```python
from build123d import *

# Parameters (mm, degrees)
SKETCH1_W           = 50.8
SKETCH1_H           = 65.000000038
SKETCH1_R           = 2.5
EXTRUDE_5_DEPTH     = 7.5
SKETCH1_3_W         = 50.8
SKETCH1_3_H         = 10
BOSS_EXTRUDE1_DEPTH = 34.125
BOSS_EXTRUDE2_START = 34.125
BOSS_EXTRUDE2_DEPTH = 5
CHAMFER1_SIZE       = 10
CHAMFER1_SIZE2      = 27.474774195
FILLET1_R           = 3
SKETCH2_R           = 5
CUT_EXTRUDE1_DEPTH  = 144.721138443
SKETCH3_R           = 2.5
CUT_EXTRUDE2_DEPTH  = 144.721138443
SKETCH4_R           = 3.55
CUT_EXTRUDE3_DEPTH  = 4
SKETCH5_R           = 3.55
CUT_EXTRUDE4_DEPTH  = 4
BOSS_EXTRUDE3_START = -3.18
SKETCH1_5_W         = 50.8
SKETCH1_5_H         = 10
SKETCH1_5_H_2       = 65.000000038
SKETCH1_5_R         = 2.5
BOSS_EXTRUDE3_DEPTH = 3.18


with BuildPart() as part:
    # Sketch1 → 5 (new body)
    with BuildSketch(Plane.XY):
        with Locations((0, 102.500000019)):
            Rectangle(SKETCH1_W, SKETCH1_H)
        with Locations((-11.25, 85.000000038)):
            Circle(SKETCH1_R, mode=Mode.SUBTRACT)
        with Locations((-11.25, 120.000000038)):
            Circle(SKETCH1_R, mode=Mode.SUBTRACT)
        with Locations((11.25, 85.000000038)):
            Circle(SKETCH1_R, mode=Mode.SUBTRACT)
        with Locations((11.25, 120.000000038)):
            Circle(SKETCH1_R, mode=Mode.SUBTRACT)
    extrude(amount=EXTRUDE_5_DEPTH)

    # Sketch1<3> → Boss-Extrude1 (add)
    with BuildSketch(Plane.XY):
        with Locations((0, 65)):
            Rectangle(SKETCH1_3_W, SKETCH1_3_H)
    extrude(amount=BOSS_EXTRUDE1_DEPTH)

    # Sketch1<4> → Boss-Extrude2 (add)
    with BuildSketch(Plane.XY.offset(BOSS_EXTRUDE2_START)):
        with BuildLine():
            Line((-25.4, 70), (-25.4, 60))
            Line((-25.4, 60), (-26, 60))
            ThreePointArc((-26, 60), (-28.828427125, 58.828427125), (-30, 56))
            Line((-30, 56), (-30, 4))
            ThreePointArc((-30, 4), (-28.828427125, 1.171572875), (-26, 0))
            Line((-26, 0), (26, 0))
            ThreePointArc((26, 0), (28.828427125, 1.171572875), (30, 4))
            Line((30, 4), (30, 56))
            ThreePointArc((30, 56), (28.828427125, 58.828427125), (26, 60))
            Line((26, 60), (25.4, 60))
            Line((25.4, 60), (25.4, 70))
            Line((25.4, 70), (-25.4, 70))
        make_face()
    extrude(amount=BOSS_EXTRUDE2_DEPTH)

    # Chamfer1
    chamfer1_edges = [part.edges().sort_by_distance(p)[0] for p in [
        (0, 70, 7.5),
    ]]
    chamfer1_side = [part.faces().sort_by_distance(p)[0] for p in [
        (0, 102.500000019, 7.5),
    ]]
    chamfer(chamfer1_edges, length=CHAMFER1_SIZE, length2=CHAMFER1_SIZE2, reference=chamfer1_side[0])

    # Fillet1
    fillet1_edges = [part.edges().sort_by_distance(p)[0] for p in [
        (0, 70, 39.125),
        (0, 70, 34.974774195),
    ]]
    fillet(fillet1_edges, radius=FILLET1_R)

    # Sketch2 → Cut-Extrude1 (cut, through all)
    with BuildSketch(Plane.XY.offset(39.125)):
        with Locations((0, 30)):
            Circle(SKETCH2_R)
    extrude(amount=-CUT_EXTRUDE1_DEPTH, mode=Mode.SUBTRACT)

    # Sketch3 → Cut-Extrude2 (cut, through all)
    with BuildSketch(Plane.XY.offset(39.125)):
        with Locations((-22.552622899, 21.79151656)):
            Circle(SKETCH3_R)
        with Locations((4.167556264, 53.635386072)):
            Circle(SKETCH3_R)
        with Locations((18.385066635, 14.573097368)):
            Circle(SKETCH3_R)
    extrude(amount=-CUT_EXTRUDE2_DEPTH, mode=Mode.SUBTRACT)

    # Sketch4 → Cut-Extrude3 (cut)
    with BuildSketch(Plane.XY.offset(39.125)):
        with Locations((4.167556264, 53.635386072)):
            Circle(SKETCH4_R)
        with Locations((-22.552622899, 21.79151656)):
            Circle(SKETCH4_R)
        with Locations((18.385066635, 14.573097368)):
            Circle(SKETCH4_R)
    extrude(amount=-CUT_EXTRUDE3_DEPTH, mode=Mode.SUBTRACT)

    # Sketch5 → Cut-Extrude4 (cut)
    with BuildSketch(Plane.XY.offset(7.5)):
        with Locations((-11.25, 120.000000038)):
            Circle(SKETCH5_R)
        with Locations((11.25, 120.000000038)):
            Circle(SKETCH5_R)
        with Locations((-11.25, 85.000000038)):
            Circle(SKETCH5_R)
        with Locations((11.25, 85.000000038)):
            Circle(SKETCH5_R)
    extrude(amount=-CUT_EXTRUDE4_DEPTH, mode=Mode.SUBTRACT)

    # Sketch1<5> → Boss-Extrude3 (add)
    # profile 1 of 2: a face of its own
    with BuildSketch(Plane.XY.offset(BOSS_EXTRUDE3_START)):
        with Locations((0, 65)):
            Rectangle(SKETCH1_5_W, SKETCH1_5_H)
    # profile 2 of 2: a face of its own
    with BuildSketch(Plane.XY.offset(BOSS_EXTRUDE3_START)):
        with Locations((0, 102.500000019)):
            Rectangle(SKETCH1_5_W, SKETCH1_5_H_2)
        with Locations((-11.25, 85.000000038)):
            Circle(SKETCH1_5_R, mode=Mode.SUBTRACT)
        with Locations((-11.25, 120.000000038)):
            Circle(SKETCH1_5_R, mode=Mode.SUBTRACT)
        with Locations((11.25, 85.000000038)):
            Circle(SKETCH1_5_R, mode=Mode.SUBTRACT)
        with Locations((11.25, 120.000000038)):
            Circle(SKETCH1_5_R, mode=Mode.SUBTRACT)
    extrude(amount=BOSS_EXTRUDE3_DEPTH)


solid = part.part
```
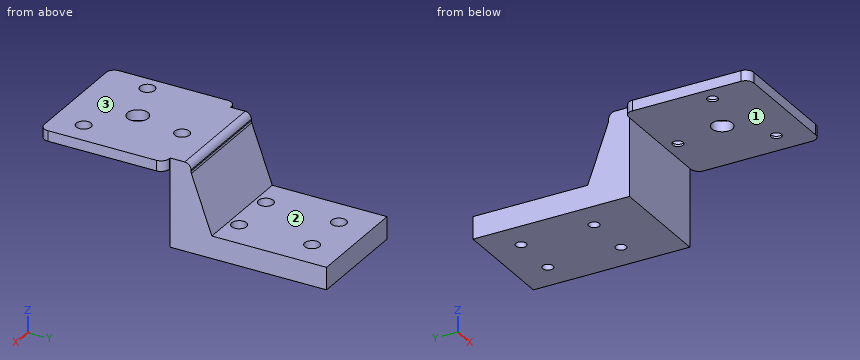
Verification items for the finished model (mm, model axes). Face numbers are marked on the shaded views. A direction names the side the tool comes from. Round coordinates to 2 decimals unless told otherwise and drop trailing zeros. Order: outer loops, then holes, each group sorted by start corner. A loop starts at its lowest first (then second) coordinate and runs counter-clockwise, first axis right, second up. Notation, with made-up numbers: (36.5, 26) -> (64.5, 26) arc R32 cw to (64.5, 61) -> close; hole circle Ø4 at (10.5, 61). An arc over 180 degrees is marked (long way). Put each result on its own line as item: value. Start each with the question number.
(1) Section check B-B (x = 11.25). Enter the section's corners in (y, z) (3 decimals), then the cut area to 3 significant figures.
(2) Section check C-C (z = 1.5). Enter the section's corners in (x, y).
(3) Tool access check on the marked faces 1, 2 and 3. Record the directions out of +Z, -Z, +X, -X, +Y, -Y that give a thin tool (end or side, any length) a straight path to the whole face; none if there is none.
(4) Material ranges on line 1 along Y through (x, z) = (-11, 1); line 2 along Y through (x, z) = (-9, 2.5); line 3 along Y through (x, z) = (0, 36), recorded low to high.
(5) Section check D-D (y = 30). Enter the section's corners in (x, z) (3 decimals), then the cut area to 3 significant figures.
(6) Depth check by flat-ended pin: pin 1 Ø5.5 at (x, y) = (18, 14.5) entering from +Z (3 decimals); pin 2 Ø4 at (x, z) = (15, 12) entering from +Y; pin 3 Ø6 at (y, z) = (120.5, 13) entering from +X; pin 4 Ø21 at (y, z) = (113, 11) entering from +X. Enter the tip coordinate at first touch or a pass-through.
(7) Section check A-A (y = 120). Enter the section's corners in (x, z).
Completed:
1. outline: (0, 34.125) -> (60, 34.125) -> (60, -3.18) -> (82.5, -3.18) -> (82.5, 3.5) -> (81.45, 3.5) -> (81.45, 7.5) -> (80, 7.5) -> (70.181, 34.478) arc R3 cw to (70, 35.504) -> (70, 36.125) arc R3 ccw to (67, 39.125) -> (0, 39.125) -> close; (87.5, -3.18) -> (117.5, -3.18) -> (117.5, 3.5) -> (116.45, 3.5) -> (116.45, 7.5) -> (88.55, 7.5) -> (88.55, 3.5) -> (87.5, 3.5) -> close; (122.5, -3.18) -> (135, -3.18) -> (135, 7.5) -> (123.55, 7.5) -> (123.55, 3.5) -> (122.5, 3.5) -> close
1. area: 1,430 mm2
2. outline: (-25.4, 60) -> (25.4, 60) -> (25.4, 135) -> (-25.4, 135) -> close; hole circle Ø5 at (-11.25, 85); hole circle Ø5 at (-11.25, 120); hole circle Ø5 at (11.25, 85); hole circle Ø5 at (11.25, 120)
3. face 1: -Z, +X, -X, -Y
3. face 2: +Z, +X, -X, +Y
3. face 3: +Z, +X, -X, +Y, -Y
4. line 1: y = 60 to 82.51, 87.49 to 117.51, 122.49 to 135
4. line 2: y = 60 to 83.91, 86.09 to 118.91, 121.09 to 135
4. line 3: y = 0 to 25, 35 to 70
5. outline: (-30, 34.125) -> (-5, 34.125) -> (-5, 39.125) -> (-30, 39.125) -> close; (5, 34.125) -> (30, 34.125) -> (30, 39.125) -> (5, 39.125) -> close
5. area: 250 mm2
6. pin 1: stops at z = 35.125
6. pin 2: stops at y = 79.09
6. pin 3: passes through
6. pin 4: stops at x = 25.4
7. outline: (-25.4, -3.18) -> (-13.75, -3.18) -> (-13.75, 3.5) -> (-14.8, 3.5) -> (-14.8, 7.5) -> (-25.4, 7.5) -> close; (-8.75, -3.18) -> (8.75, -3.18) -> (8.75, 3.5) -> (7.7, 3.5) -> (7.7, 7.5) -> (-7.7, 7.5) -> (-7.7, 3.5) -> (-8.75, 3.5) -> close; (13.75, -3.18) -> (25.4, -3.18) -> (25.4, 7.5) -> (14.8, 7.5) -> (14.8, 3.5) -> (13.75, 3.5) -> close
